```python
from build123d import *

# Parameters (mm, degrees)
F0_W     = 150
F0_H     = 75
F1_DEPTH = 5
F3_DEPTH = 5.001
F5_DEPTH = 5.001
F6_W     = 50
F6_H     = 25
F7_DEPTH = 5.001
F8_R     = 4.99999


# Not quite as in the source:
# - a fillet or chamfer is up to 0.001 mm smaller than in the source, because OpenCascade refuses the exact size


with BuildPart() as f1:
    # F0 (on Top) → F1 (new body)
    with BuildSketch(Plane.XY):
        with Locations((75, 37.5)):
            Rectangle(F0_W, F0_H)
    extrude(amount=F1_DEPTH)

    # F2 (on face) → F3 (cut, through all)
    with BuildSketch(Plane.XY.offset(5)):
        with BuildLine():
            Line((13, 40), (13, 0))
            Line((13, 0), (27, 0))
            Line((27, 0), (27, 40))
            ThreePointArc((27, 40), (20, 47), (13, 40))
        make_face()
    extrude(amount=-F3_DEPTH, mode=Mode.SUBTRACT)

    # F4 (on face) → F5 (cut, through all)
    with BuildSketch(Plane.XY.offset(5)):
        with BuildLine():
            Line((137, 35), (137, 75))
            Line((137, 75), (123, 75))
            Line((123, 75), (123, 35))
            ThreePointArc((123, 35), (130, 28), (137, 35))
        make_face()
    extrude(amount=-F5_DEPTH, mode=Mode.SUBTRACT)

    # F6 (on face) → F7 (cut, through all)
    with BuildSketch(Plane.XY.offset(5)):
        with Locations((71.2950700867, 37.5)):
            Rectangle(F6_W, F6_H)
    extrude(amount=-F7_DEPTH, mode=Mode.SUBTRACT)

    # F8 (radius 5 in the source; OpenCascade refuses exactly that, so slightly less here)
    f8_edges = [f1.edges().sort_by_distance(p)[0] for p in [
        (88.5, 0, 5),
        (27, 20, 5),
        (150, 37.5, 5),
        (20, 47, 5),
        (143.5, 75, 5),
        (13, 20, 5),
        (137, 55, 5),
        (6.5, 0, 5),
        (130, 28, 5),
        (0, 37.5, 5),
        (123, 55, 5),
        (61.5, 75, 5),
        (71.29507, 50, 5),
        (46.29507, 37.5, 5),
        (71.29507, 25, 5),
        (96.29507, 37.5, 5),
    ]]
    fillet(f8_edges, radius=F8_R)


solid = f1.part
```
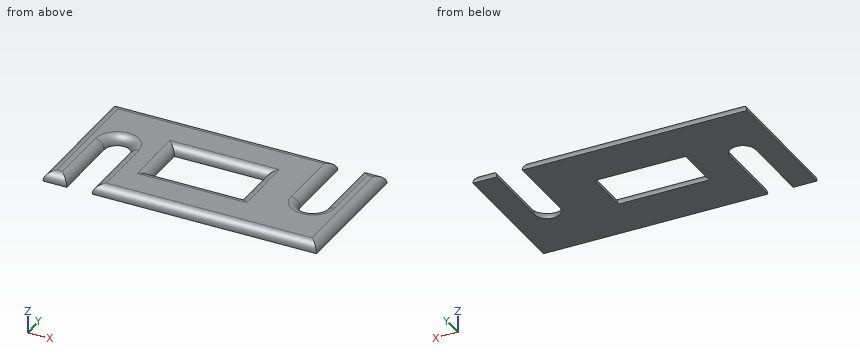
Work out the finished part from the listing and answer in its coordinate system (mm). Coordinates: 2 decimals unless noted, no trailing zeros. Write each loop counter-clockwise with the first axis right and the second up, starting at its lowest first coordinate (ties: lowest second). Pieces come first, ordered by that corner, then holes.
Q1. A cutting plane is placed at D-D, the plane z = 2.9. Give the vertices of the cut face in (x, y).
Q2. Find the intervals of material crossed by line 1 (X direction, y = 45.5, z = 3.65); line 2 (X direction, y = 49, z = 2.1); line 3 (Y direction, x = 141, z = 0.55), in increasing order.
Q3. Each of these flat-tipped pins is pushed along its axis until it touches: pin 1 Ø8 at (x, y) = (100, 13.5) entering from -Z; pin 2 Ø2 at (y, z) = (15.5, 4) entering from +X. Where does it stop, or does it pass through?
Findings below:
1. outline: (0.93, 0.93) - (12.07, 0.93) - (12.07, 40) arc R7.93 cw to (27.93, 40) - (27.93, 0.93) - (149.07, 0.93) - (149.07, 74.07) - (137.93, 74.07) - (137.93, 35) arc R7.93 cw to (122.07, 35) - (122.07, 74.07) - (0.93, 74.07) - close; hole (45.37, 24.07) - (97.22, 24.07) - (97.22, 50.93) - (45.37, 50.93) - close
2. line 1: x = 1.58 to 13.41, 26.59 to 44.71, 97.88 to 121.42, 138.58 to 148.42
2. line 2: x = 0.46 to 45.83, 96.76 to 122.54, 137.46 to 149.54
2. line 3: y = 0.03 to 74.97
3. pin 1: stops at z = 0
3. pin 2: stops at x = 149
